For this review, take the finished solid that the model builds, in its own axes (mm). A direction names the side the tool comes from. Give positions to 0.01 mm unless a question says otherwise; leave off trailing zeros. Loops run counter-clockwise (first coordinate to the right, second up) from the corner with the lowest first, then second, coordinate; pieces in that order, holes last. Notation, with made-up numbers: (1.5, 37.5) -> (31.5, 37.5) arc R10 ccw to (31.5, 49.5) -> close; hole circle Ø5 at (71.5, 29.25). An arc over 180 degrees is marked (long way). One line per question, with ' | ' between items. Start each with the question number.
(1) Draft analysis for pull direction X (two halves, no side actions). For faces 1 (the flat face through (-78, 119, 72)), 2 (the cylindrical face through (-76.76, 120.5, 36.5)), 3 (the flat face through (-78, 121, 150.6)), 4 (the cylindrical face through (-77.52, 116.34, 74.25)), state which applies: +X half, -X half, draft (parallel to the pull), parting line (faces both ways), or undercut.
(2) Wall thickness on probe 1 along Y at (x, z) = (-77.65, 99); probe 2 along X at (y, z) = (119.05, 127.5); probe 3 along Z at (x, y) = (-79.35, 119.35): over which ranges is each line inside the solid? List them lowest first.
(3) Tool access review of faces 5 (the flat face through (-78, 121, 0)), 6 (the flat face through (-78, 119, 78.6)): name each direction out of +Z, -Z, +X, -X, +Y, -Y from which nothing blocks a thin tool from reaching the whole face with its end or side.
(4) Consider section A-A (z = 14). Write out the cut boundary in (x, y) (3 decimals), and give its area (3 significant figures).
(5) Insertion check: P1, Ø1.1, axis at x = -78.5, y = 119, coming from the +Z side. The pin has a flat end and moves straight along its axis. Give the tip position at first contact, or say it passes through.
from build123d import *

# Parameters (mm, degrees)
SALIENTE_EXTRUIR1_DEPTH = 150.6
CROQUIS2_R              = 1.875
CORTAR_EXTRUIR1_DEPTH   = 72
CORTAR_EXTRUIR2_START   = -72
CROQUIS3_R              = 1.875
CORTAR_EXTRUIR2_DEPTH   = 72


with BuildPart() as part:
    # Croquis1 → Saliente-Extruir1 (new body)
    with BuildSketch(Plane.XY):
        with BuildLine():
            Line((-78.077598734, 121.298692457), (-78.077598734, 121.898692457))
            Line((-78.077598734, 121.898692457), (-77.177598734, 121.898692457))
            Line((-77.177598734, 121.898692457), (-77.177598734, 121.298692457))
            ThreePointArc((-77.177598734, 121.298692457), (-77.627598734, 116.339525931), (-78.077598734, 121.298692457))
        make_face()
    extrude(amount=SALIENTE_EXTRUIR1_DEPTH)

    # Croquis2 → Cortar-Extruir1 (cut)
    with BuildSketch(Plane.XY.offset(150.6)):
        with Locations((-77.627598734, 118.839525931)):
            Circle(CROQUIS2_R)
    extrude(amount=-CORTAR_EXTRUIR1_DEPTH, mode=Mode.SUBTRACT)

    # Croquis3 → Cortar-Extruir2 (cut)
    with BuildSketch(Plane(origin=(0, 0, 0), x_dir=(-1, 0, 0), z_dir=(0, 0, -1)).offset(CORTAR_EXTRUIR2_START)):
        with Locations(Location((77.627598734, 118.839525931, 0), (0, 0, 180))):
            Circle(CROQUIS3_R)
    extrude(amount=CORTAR_EXTRUIR2_DEPTH, mode=Mode.SUBTRACT)


solid = part.part
A:
1) face 1: undercut | face 2: undercut | face 3: draft | face 4: parting line
2) probe 1: y = 116.34 to 116.96, 120.71 to 121.9 | probe 2: x = -80.12 to -79.49, -75.76 to -75.14 | probe 3: z = 72 to 78.6
3) face 5: -Z, +X, -X, +Y, -Y | face 6: +Z
4) outline: (-78.078, 121.299) arc R2.5 ccw (long way) to (-77.178, 121.299) -> (-77.178, 121.899) -> (-78.078, 121.899) -> close; hole circle Ø3.75 at (-77.628, 118.84) | area: 9.11 mm^2
5) P1: stops at z = 78.6
